from build123d import *

# Parameters (mm, degrees)
SKETCH1_R           = 1.75
BOSS_EXTRUDE1_DEPTH = 10
SKETCH2_R           = 2.5
CUT_EXTRUDE1_DEPTH  = 51.644943511
BOSS_EXTRUDE2_DEPTH = 12
SKETCH4_R           = 2
CUT_EXTRUDE2_DEPTH  = 25


with BuildPart() as part:
    # Sketch1 → Boss-Extrude1 (new body)
    with BuildSketch(Plane(origin=(0, 0, 0), x_dir=(1, 0, 0), z_dir=(0, 1, 0))):
        with BuildLine():
            Line((-5, 0), (-5, 43.630343442))
            ThreePointArc((-5, 43.630343442), (0, 48.630343442), (5, 43.630343442))
            Line((5, 43.630343442), (5, 11))
            ThreePointArc((5, 11), (4, 10), (5, 9))
            Line((5, 9), (5, 0))
            ThreePointArc((5, 0), (0, -5), (-5, 0))
        make_face()
        with Locations(Location((0, 0, 0), (0, 0, 270))):
            Circle(SKETCH1_R, mode=Mode.SUBTRACT)
        with Locations(Location((0, 25, 0), (0, 0, 270))):
            Circle(SKETCH1_R, mode=Mode.SUBTRACT)
        with Locations(Location((0, 35, 0), (0, 0, 270))):
            Circle(SKETCH1_R, mode=Mode.SUBTRACT)
    extrude(amount=BOSS_EXTRUDE1_DEPTH)

    # Sketch2 → Cut-Extrude1 (cut, through all)
    with BuildSketch(Plane(origin=(5, 0, 0), x_dir=(0, 0, -1), z_dir=(1, 0, 0))):
        with Locations((20, 5)):
            Circle(SKETCH2_R)
    extrude(amount=-CUT_EXTRUDE1_DEPTH, mode=Mode.SUBTRACT)

    # Sketch3 → Boss-Extrude2 (add)
    with BuildSketch(Plane(origin=(0, 10, 0), x_dir=(1, 0, 0), z_dir=(0, 1, 0))):
        with BuildLine():
            Line((5, 5.5), (-5, 5.5))
            Line((-5, 5.5), (-5, 18))
            Line((-5, 18), (5, 18))
            Line((5, 18), (5, 11))
            ThreePointArc((5, 11), (4, 10), (5, 9))
            Line((5, 9), (5, 5.5))
        make_face()
    extrude(amount=BOSS_EXTRUDE2_DEPTH)

    # Sketch4 → Cut-Extrude2 (cut)
    with BuildSketch(Plane.XY.offset(-55)):
        with Locations(Location((0, 5, 0), (0, 0, 180))):
            Circle(SKETCH4_R)
    extrude(amount=CUT_EXTRUDE2_DEPTH, mode=Mode.SUBTRACT)


solid = part.part
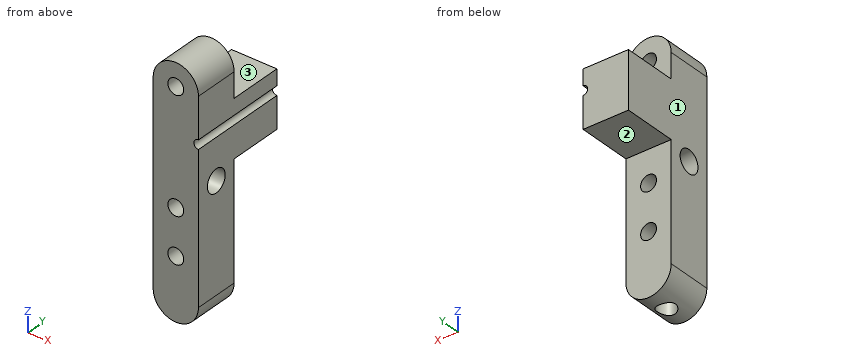
The listing builds one solid part. Answer for the finished solid, in the listing's coordinates (mm). Face numbers are marked on the shaded views. A direction names the side the tool comes from. Coordinates: 2 decimals unless noted, no trailing zeros. Write each loop counter-clockwise with the first axis right and the second up, starting at its lowest first coordinate (ties: lowest second). Pieces come first, ordered by that corner, then holes. Notation, with made-up numbers: M 89.5,21.5 L 147.5,21.5 A16 ccw 147.5,44.5 Z; hole C 36,12 d5. An arc over 180 degrees is marked long. Write each question's results on one line, items separated by ' | '.
Item 1: The part is cut by section D-D on x = -4. Determine the outline of the cut face in (y, z), and give its area (3 significant figures).
Answer below:
outline: M 0,-46.63 L 10,-46.63 L 10,-18 L 22,-18 L 22,-5.5 L 10,-5.5 L 10,3 L 0,3 Z; hole C 5,-20 d5 | area: 627 mm2
Item 2: Given P1, Ø1.5, axis at x = 3, y = 14, coming from the -Z side; P2, Ø2, axis at x = -2, y = 4, coming from the +Z side; P3, Ø2, axis at x = 0, z = -35, coming from the +Y side; P4, Ø3, axis at x = 0.5, y = 5.5, coming from the -Z side, each flat-ended and moving along its own axis, determine where each tip first touches the part or whether it passes through.
Answer below:
P1: z = -18 | P2: z = 4.9 | P3: through | P4: z = -48.62
Item 3: The part is cut by section A-A on z = -20. Determine the outline of the cut face in (x, y), and give its area (3 significant figures).
Answer below:
outline: M -5,0 L 5,0 L 5,2.5 L -5,2.5 Z; M -5,7.5 L 5,7.5 L 5,10 L -5,10 Z | area: 50.0 mm2
Item 4: Consider probe 1 along X at (y, z) = (5.25, -25); probe 2 along Z at (x, y) = (-2, 14.5); probe 3 along Y at (x, z) = (3.25, 0). Determine where each line is inside the solid, lowest interval first. Write a range as [from, to].
Answer below:
probe 1: [-5, -1.75], [1.75, 5] | probe 2: [-18, -5.5] | probe 3: [0, 10]
Item 5: The part is cut by section B-B on x = 0. State how many separate pieces and enclosed holes the cut face has, and give its area (3 significant figures).
Answer below:
separate pieces: 5 | enclosed holes: 1 | area: 501 mm2
Item 6: The part is cut by section C-C on y = 13.25. Determine the outline of the cut face in (x, z), and give its area (3 significant figures).
Answer below:
outline: M -5,-18 L 5,-18 L 5,-11 A1 cw 5,-9 L 5,-5.5 L -5,-5.5 Z | area: 123 mm2
Item 7: Which of the six approach directions +Z, -Z, +X, -X, +Y, -Y give full straight-line access (tool end or side, diameter ignored) to the marked faces 1, 2 and 3?
Answer below:
face 1: +Z, -Z, -X, +Y, -Y | face 2: -Z, +X, -X, +Y | face 3: +Z, +X, -X, +Y
